Geometry: see drawing. Coordinates: mm, zero at the bounding-box minimum. Coordinates: 2 decimals unless noted, no trailing zeros. Loops run counter-clockwise (first coordinate to the right, second up) from the corner with the lowest first, then second, coordinate; pieces in that order, holes last. Notation, with made-up numbers: (68.25, -3.75) - (123.25, -3.75) arc R10 ccw to (123.25, 1.25) - close; hole circle Ø4 at (85.5, -7.75). An arc over 180 degrees is marked (long way). Answer in a Markdown table with one row per item.
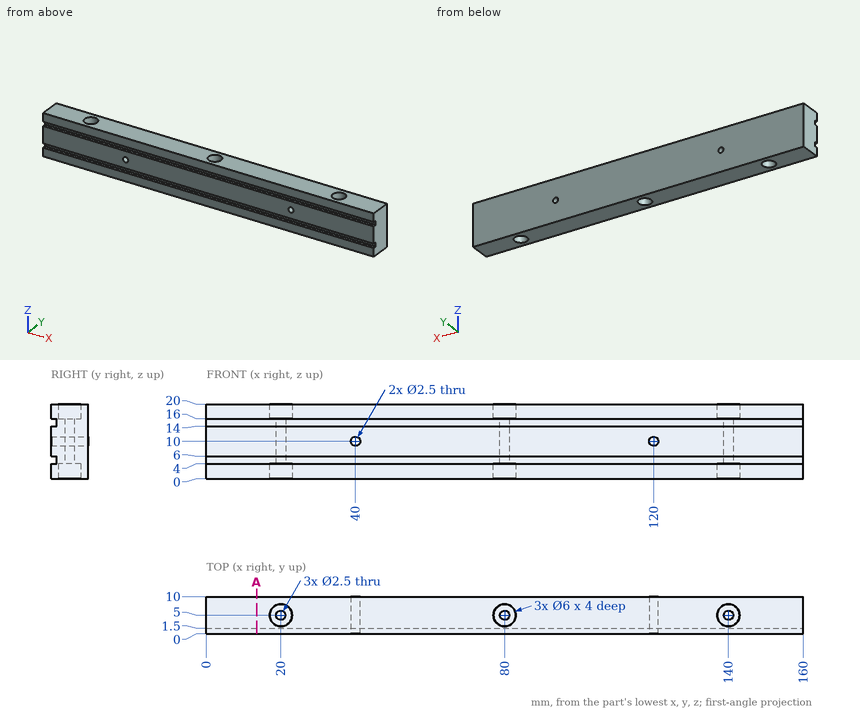
(1) Ray query, probe 1 along Y at (x, z) = (140, 1.9); probe 2 along X at (y, z) = (5, 18.2); probe 3 along X at (y, z) = (3.5, 11). Return the intervals inside material, ascending.
Verdict:
| item | result |
|---|---|
| probe 1 | y = 0 to 2, 8 to 10 |
| probe 2 | x = 0 to 17, 23 to 77, 83 to 137, 143 to 160 |
| probe 3 | x = 0 to 39.25, 40.75 to 119.25, 120.75 to 160 |
(2) First-contact query: pin 1 Ø3 at (x, y) = (18, 6.5) entering from -Z; pin 2 Ø5.5 at (x, y) = (140, 5) entering from -Z; pin 3 Ø1 at (x, z) = (103, 5) entering from -Y; pin 4 Ø5.5 at (x, y) = (80, 5) entering from +Z. Flat tips, straight axial feed; report the tip coordinate or a pass-through.
Verdict:
| item | result |
|---|---|
| pin 1 | stops at z = 0 |
| pin 2 | stops at z = 4 |
| pin 3 | stops at y = 1.5 |
| pin 4 | stops at z = 16 |
(3) Cut plane A-A on x = 13.5. Output: boundary loops of the cut face in (y, z), then the cut area to 3 significant figures.
Verdict:
| item | result |
|---|---|
| outline | (0, 0) - (10, 0) - (10, 20) - (0, 20) - (0, 16) - (1.5, 16) - (1.5, 14) - (0, 14) - (0, 6) - (1.5, 6) - (1.5, 4) - (0, 4) - close |
| area | 194 mm² |
